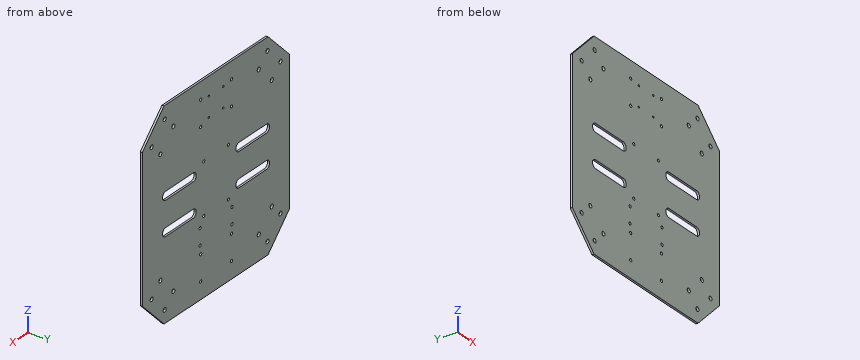
from build123d import *

# Parameters (mm, degrees)
BOSS_EXTRUDE1_DEPTH = 3.175
SKETCH2_R           = 3.175
CUT_EXTRUDE1_DEPTH  = 6.35
SKETCH3_R           = 2.159
CUT_EXTRUDE2_DEPTH  = 6.35
SKETCH4_R           = 2.2225
CUT_EXTRUDE3_DEPTH  = 351.937720963
SKETCH10_R          = 1.397
CUT_EXTRUDE4_DEPTH  = 351.937720963
SKETCH11_R          = 2.159
CUT_EXTRUDE6_DEPTH  = 351.937720963


with BuildPart() as part:
    # Sketch1 → Boss-Extrude1 (new body)
    with BuildSketch(Plane(origin=(0, 0, 0), x_dir=(1, 0, 0), z_dir=(0, 1, 0))):
        Polygon((-16.864769233, 51.656360067), (-61.766049839, 6.755079462), (-61.766049839, -208.242359328), (-16.864769233, -253.143639933), (198.132669556, -253.143639933), (243.033950161, -208.242359328), (243.033950161, 6.755079462), (198.132669556, 51.656360067), align=None)
        with BuildLine():
            ThreePointArc((43.337601054, -119.793639933), (49.687601054, -126.143639933), (43.337601054, -132.493639933))
            Line((43.337601054, -132.493639933), (-13.679235779, -132.493639933))
            ThreePointArc((-13.679235779, -132.493639933), (-20.029235779, -126.143639933), (-13.679235779, -119.793639933))
            Line((-13.679235779, -119.793639933), (43.337601054, -119.793639933))
        make_face(mode=Mode.SUBTRACT)
        with BuildLine():
            Line((194.947136102, -132.493639933), (137.930299269, -132.493639933))
            ThreePointArc((137.930299269, -132.493639933), (131.580299269, -126.143639933), (137.930299269, -119.793639933))
            Line((137.930299269, -119.793639933), (194.947136102, -119.793639933))
            ThreePointArc((194.947136102, -119.793639933), (201.297136102, -126.143639933), (194.947136102, -132.493639933))
        make_face(mode=Mode.SUBTRACT)
        with BuildLine():
            Line((-13.679235779, -68.993639933), (43.337601054, -68.993639933))
            ThreePointArc((43.337601054, -68.993639933), (49.687601054, -75.343639933), (43.337601054, -81.693639933))
            Line((43.337601054, -81.693639933), (-13.679235779, -81.693639933))
            ThreePointArc((-13.679235779, -81.693639933), (-20.029235779, -75.343639933), (-13.679235779, -68.993639933))
        make_face(mode=Mode.SUBTRACT)
        with BuildLine():
            ThreePointArc((137.930299269, -81.693639933), (131.580299269, -75.343639933), (137.930299269, -68.993639933))
            Line((137.930299269, -68.993639933), (194.947136102, -68.993639933))
            ThreePointArc((194.947136102, -68.993639933), (201.297136102, -75.343639933), (194.947136102, -81.693639933))
            Line((194.947136102, -81.693639933), (137.930299269, -81.693639933))
        make_face(mode=Mode.SUBTRACT)
    extrude(amount=BOSS_EXTRUDE1_DEPTH)

    # Sketch2 → Cut-Extrude1 (cut)
    with BuildSketch(Plane(origin=(0, 3.175, 0), x_dir=(1, 0, 0), z_dir=(0, 1, 0))):
        with Locations(Location((-15.627316695, 32.458395287, 0), (0, 0, 270))):
            Circle(SKETCH2_R)
        with Locations(Location((2.333195547, 14.497883045, 0), (0, 0, 270))):
            Circle(SKETCH2_R)
        with Locations(Location((-24.607572816, -12.442885319, 0), (0, 0, 270))):
            Circle(SKETCH2_R)
        with Locations(Location((-42.568085059, 5.517626924, 0), (0, 0, 270))):
            Circle(SKETCH2_R)
        with Locations(Location((205.875473139, -12.442885319, 0), (0, 0, 270))):
            Circle(SKETCH2_R)
        with Locations(Location((223.835985381, 5.517626924, 0), (0, 0, 270))):
            Circle(SKETCH2_R)
        with Locations(Location((178.934704776, 14.497883045, 0), (0, 0, 270))):
            Circle(SKETCH2_R)
        with Locations(Location((196.895217018, 32.458395287, 0), (0, 0, 270))):
            Circle(SKETCH2_R)
        with Locations(Location((-24.607572816, -189.044394548, 0), (0, 0, 270))):
            Circle(SKETCH2_R)
        with Locations(Location((-42.568085059, -207.00490679, 0), (0, 0, 270))):
            Circle(SKETCH2_R)
        with Locations(Location((-15.627316695, -233.945675153, 0), (0, 0, 270))):
            Circle(SKETCH2_R)
        with Locations(Location((2.333195547, -215.985162911, 0), (0, 0, 270))):
            Circle(SKETCH2_R)
        with Locations(Location((223.835985381, -207.00490679, 0), (0, 0, 270))):
            Circle(SKETCH2_R)
        with Locations(Location((196.895217018, -233.945675153, 0), (0, 0, 270))):
            Circle(SKETCH2_R)
        with Locations(Location((178.934704776, -215.985162911, 0), (0, 0, 270))):
            Circle(SKETCH2_R)
        with Locations(Location((205.875473139, -189.044394548, 0), (0, 0, 270))):
            Circle(SKETCH2_R)
    extrude(amount=-CUT_EXTRUDE1_DEPTH, mode=Mode.SUBTRACT)

    # Sketch3 → Cut-Extrude2 (cut)
    with BuildSketch(Plane(origin=(0, 3.175, 0), x_dir=(1, 0, 0), z_dir=(0, 1, 0))):
        with Locations(Location((65.233950161, -62.643639933, 0), (0, 0, 270))):
            Circle(SKETCH3_R)
        with Locations(Location((116.033950161, -62.643639933, 0), (0, 0, 270))):
            Circle(SKETCH3_R)
        with Locations(Location((65.233950161, -138.843639933, 0), (0, 0, 270))):
            Circle(SKETCH3_R)
        with Locations(Location((116.033950161, -138.843639933, 0), (0, 0, 270))):
            Circle(SKETCH3_R)
    extrude(amount=-CUT_EXTRUDE2_DEPTH, mode=Mode.SUBTRACT)

    # Sketch4 → Cut-Extrude3 (cut, through all)
    with BuildSketch(Plane(origin=(0, 3.175, 0), x_dir=(1, 0, 0), z_dir=(0, 1, 0))):
        with Locations(Location((58.883950161, 26.256360067, 0), (0, 0, 270))):
            Circle(SKETCH4_R)
        with Locations(Location((122.383950161, 26.256360067, 0), (0, 0, 270))):
            Circle(SKETCH4_R)
        with Locations(Location((58.883950161, -11.843639933, 0), (0, 0, 270))):
            Circle(SKETCH4_R)
        with Locations(Location((122.383950161, -11.843639933, 0), (0, 0, 270))):
            Circle(SKETCH4_R)
        with Locations(Location((122.383950161, -189.643639933, 0), (0, 0, 90))):
            Circle(SKETCH4_R)
        with Locations(Location((58.883950161, -189.643639933, 0), (0, 0, 90))):
            Circle(SKETCH4_R)
        with Locations(Location((122.383950161, -227.743639933, 0), (0, 0, 90))):
            Circle(SKETCH4_R)
        with Locations(Location((58.883950161, -227.743639933, 0), (0, 0, 90))):
            Circle(SKETCH4_R)
    extrude(amount=-CUT_EXTRUDE3_DEPTH, mode=Mode.SUBTRACT)

    # Sketch10 → Cut-Extrude4 (cut, through all)
    with BuildSketch(Plane(origin=(0, 0, 0), x_dir=(-1, 0, 0), z_dir=(0, -1, 0))):
        with Locations(Location((-105.619950161, -195.222402366, 0), (0, 0, 90))):
            Circle(SKETCH10_R)
        with Locations(Location((-105.619950161, -225.194402366, 0), (0, 0, 90))):
            Circle(SKETCH10_R)
        with Locations(Location((-75.647950161, -225.194402366, 0), (0, 0, 270))):
            Circle(SKETCH10_R)
        with Locations(Location((-75.647950161, -195.222402366, 0), (0, 0, 270))):
            Circle(SKETCH10_R)
    extrude(amount=-CUT_EXTRUDE4_DEPTH, mode=Mode.SUBTRACT)

    # Sketch11 → Cut-Extrude6 (cut, through all)
    with BuildSketch(Plane.XZ):
        with Locations(Location((123.653950161, 24.543639933, 0), (0, 0, 270))):
            Circle(SKETCH11_R)
        with Locations(Location((123.653950161, 48.673639933, 0), (0, 0, 90))):
            Circle(SKETCH11_R)
        with Locations(Location((57.613950161, 48.673639933, 0), (0, 0, 270))):
            Circle(SKETCH11_R)
        with Locations(Location((57.613950161, 24.543639933, 0), (0, 0, 90))):
            Circle(SKETCH11_R)
    extrude(amount=-CUT_EXTRUDE6_DEPTH, mode=Mode.SUBTRACT)


solid = part.part
For this review, take the finished solid that the model builds, in its own axes (mm). Give positions to 0.01 mm unless a question says otherwise; leave off trailing zeros. Loops run counter-clockwise (first coordinate to the right, second up) from the corner with the lowest first, then second, coordinate; pieces in that order, holes last. Notation, with made-up numbers: M 36.5,57 L 83.5,57 A5 cw 83.5,62 Z; hole C 68,38 d5. An arc over 180 degrees is marked long. Answer as a JSON object with one key per item and string values. Group by question number.
Q1. Insertion check: P1, Ø4, axis at x = 223.84, z = 207, coming from the +Y side. The pin has a flat end and moves straight along its axis. Give the tip position at first contact, or say it passes through.
Q2. Add section B-B on y = 2.5. Give the number of separate pieces and of enclosed holes in the cut face, and give its area (3 significant figures).
Q3. For probe 1 along Z at (x, y) = (30, 2.4); probe 2 along X at (y, z) = (0.95, 49); probe 3 along X at (y, z) = (0.85, 213.5), list the stretches that pass through material, from the lowest coordinate up. Write a range as [from, to].
Q4. Add section A-A on x = 152.5. Give the boundary of the cut face in (y, z) (3 decimals).
Q5. Add section C-C on x = -33.5. Give the boundary of the cut face in (y, z) (3 decimals).
Checked values:
{
 "1": {"P1": "through"},
 "2": {"separate pieces": "1", "enclosed holes": "40", "area": "84,700 mm²"},
 "3": {"probe 1": "[-51.66, 68.99], [81.69, 119.79], [132.49, 253.14]", "probe 2": "[-61.77, 55.48], [59.75, 121.52], [125.79, 243.03]", "probe 3": "[-56.51, 0.36], [4.31, 176.96], [180.91, 237.78]"},
 "4": {"outline": "M 0,-51.656 L 3.175,-51.656 L 3.175,68.994 L 0,68.994 Z; M 0,81.694 L 3.175,81.694 L 3.175,119.794 L 0,119.794 Z; M 0,132.494 L 3.175,132.494 L 3.175,253.144 L 0,253.144 Z"},
 "5": {"outline": "M 0,-35.021 L 3.175,-35.021 L 3.175,236.508 L 0,236.508 Z"}
}
